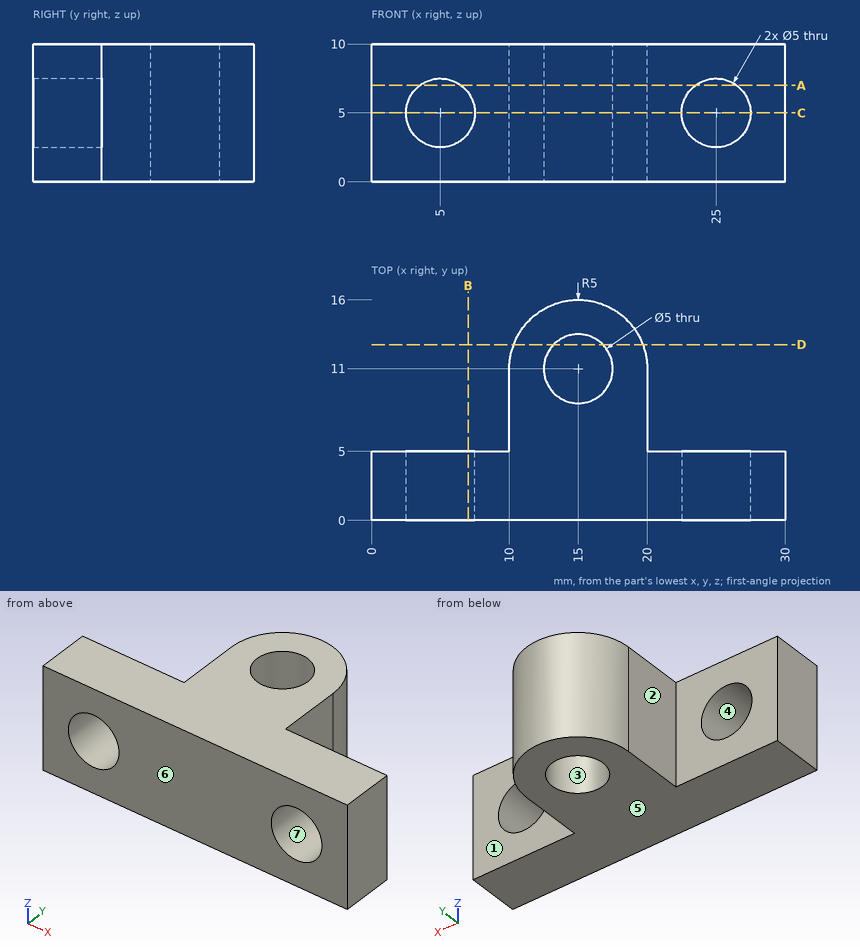
Print and shaded views of the part. All mm, measured from the part's lowest x, y and z. A direction names the side the tool comes from. Coordinates: 2 decimals unless noted, no trailing zeros. Loops run counter-clockwise (first coordinate to the right, second up) from the corner with the lowest first, then second, coordinate; pieces in that order, holes last. Notation, with made-up numbers: (6.25, 32.25) - (20.25, 32.25) arc R21 ccw to (20.25, 62.25) - close; hole circle Ø1 at (26, 74). An arc over 180 degrees is marked (long way). Use one line per item in the form item = value. Start each with the question number.
1) Drill centre lines: L1, parallel to Y at x = 15, z = 5.25; L2, parallel to Y at x = 6, z = 2; L3, parallel to X at y = 8.25, z = 1.25. Where is each one in solid material? Low to high. Write a range as from..to.
2) Tool access for the marked faces 1, 2 and 3: list every direction of +Z, -Z, +X, -X, +Y, -Y with a clear straight run to the whole face (end or side of a thin tool).
3) Band-saw the part on A-A (z = 7). Give the cut face in (x, y).
4) Two-plate mould, pull along Z, no slides. Class the marked faces 4, 5, 6 and 7: +Z half, -Z half, draft (parallel to the pull), parting line (faces both ways), or undercut.
5) Band-saw the part on D-D (y = 12.75). Give the cut face in (x, z).
6) Flat gauge pins, fed straight in: pin 1 (6 mm diameter, centred on x = 9.5, z = 3.5, fed in from -Y); pin 2 (3 mm diameter, centred on x = 7.5, z = 6, fed in from +Y); pin 3 (4 mm diameter, centred on y = 11.5, z = 2.5, fed in from -X); pin 4 (3 mm diameter, centred on y = 7.5, z = 5.5, fed in from +X). Where does each tip first touch, or does it go through?
7) Band-saw the part on B-B (x = 7). Give the cut face in (y, z), and give its area (3 significant figures).
8) Band-saw the part on C-C (z = 5). Give the cut face in (x, y).
Check values:
q1.L1 = 0..8.5, 13.5..16
q1.L2 = 0..5
q1.L3 = 10..20
q2.face_1 = +Z, -Z, +X, +Y
q2.face_2 = +Z, -Z, -X, +Y
q2.face_3 = +Z, -Z
q3.outline = (0, 0) - (3.5, 0) - (3.5, 5) - (0, 5) - close; (6.5, 0) - (23.5, 0) - (23.5, 5) - (20, 5) - (20, 11) arc R5 ccw to (10, 11) - (10, 5) - (6.5, 5) - close; (26.5, 0) - (30, 0) - (30, 5) - (26.5, 5) - close; hole circle Ø5 at (15, 11)
q4.face_4 = undercut
q4.face_5 = -Z half
q4.face_6 = draft
q4.face_7 = undercut
q5.outline = (10.32, 0) - (13.21, 0) - (13.21, 10) - (10.32, 10) - close; (16.79, 0) - (19.68, 0) - (19.68, 10) - (16.79, 10) - close
q6.pin_1 = 0
q6.pin_2 = 5
q6.pin_3 = 10
q6.pin_4 = 20
q7.outline = (0, 0) - (5, 0) - (5, 3.5) - (0, 3.5) - close; (0, 6.5) - (5, 6.5) - (5, 10) - (0, 10) - close
q7.area = 35.0 mm2
q8.outline = (0, 0) - (2.5, 0) - (2.5, 5) - (0, 5) - close; (7.5, 0) - (22.5, 0) - (22.5, 5) - (20, 5) - (20, 11) arc R5 ccw to (10, 11) - (10, 5) - (7.5, 5) - close; (27.5, 0) - (30, 0) - (30, 5) - (27.5, 5) - close; hole circle Ø5 at (15, 11)
